Model file for the job. Use its own axes, mm. A direction names the side the tool comes from. Round coordinates to 2 decimals unless told otherwise and drop trailing zeros. Order: outer loops, then holes, each group sorted by start corner. A loop starts at its lowest first (then second) coordinate and runs counter-clockwise, first axis right, second up. Notation, with made-up numbers: (53, -38.75) - (62, -38.75) arc R23 cw to (62, -14.75) - close; hole circle Ø11 at (-24, 52.5). An arc over 180 degrees is marked (long way). Answer as CSV lines item,"result". Start each with the question number.
1. Band-saw the part on A-A on x = -4.75. List the corners of the cut face in (y, z), then the cut area to 3 significant figures.
2. Pull direction Y, two halves, no side cores. Call faces 1 (the face through (10.3, -7.1, 1.4)), 2 (the face through (11.27, -5.35, 1.4)), 3 (the face through (-4.95, 8.69, 1.4)): released by +Y, released by -Y, zero draft, split by the parting line, or undercut.
3. Wall check: line 1 along Y through (x, z) = (-0.65, 80); line 2 along Z through (x, y) = (0.8, -12.5); line 3 along X through (y, z) = (-11, 52.5). Give the ranges that are in metal, low to high. Write a range as [from, to].
4. Pin check, flat tips, straight feed: pin 1 Ø2.5 at (y, z) = (-12.5, 0) entering from +X; pin 2 Ø1.6 at (y, z) = (-12.5, 40) entering from +X; pin 3 Ø4 at (x, z) = (3.5, 74.5) entering from +Y; pin 4 Ø4 at (y, z) = (12.5, 29.5) entering from -X. Stop position of each tip, or through.
5. 3-axis set-ups, long thin cutter, end or side, ignore diameter. For faces 4 (the face through (11.04, -5.796, 1.4)), 5 (the face through (11.27, 5.35, 1.4)), 6 (the face through (0.5, -12.5, 1.4)): which of +Z, -Z, +X, -X, +Y, -Y reach the whole face in a straight line?
```python
from build123d import *

# Parameters (mm, degrees)
SKETCH1_R           = 10
BOSS_EXTRUDE1_DEPTH = 100
SKETCH4_W           = 0.5
SKETCH4_H           = 15
BOSS_EXTRUDE3_DEPTH = 200
CIRPATTERN7_COUNT   = 6
SKETCH7_R           = 1
CUT_EXTRUDE2_DEPTH  = 5
CIRPATTERN9_COUNT   = 6


with BuildPart() as part:
    # Sketch1 → Boss-Extrude1 (new, symmetric)
    with BuildSketch(Plane.XY):
        Circle(SKETCH1_R)
    extrude(amount=BOSS_EXTRUDE1_DEPTH, both=True)

    # Sketch4 → Boss-Extrude3 (add)
    with BuildSketch(Plane.XY.offset(100)):
        with Locations((-0.75, 7.5)):
            Rectangle(SKETCH4_W, SKETCH4_H)
        with Locations((0.75, 7.5)):
            Rectangle(SKETCH4_W, SKETCH4_H)
    boss_extrude3 = extrude(amount=-BOSS_EXTRUDE3_DEPTH)

    # CirPattern7: Boss-Extrude3 ×6 about axis
    cirpattern7_axis = Axis((0, 0, 0), (0, 0, 1))
    for i in range(1, CIRPATTERN7_COUNT):
        add(boss_extrude3.rotate(cirpattern7_axis, i * 360 / CIRPATTERN7_COUNT))

    # Sketch7 → Cut-Extrude2 (cut)
    with BuildSketch(Plane.ZY.offset(1)):
        with Locations((-80, 12.5)):
            Circle(SKETCH7_R)
        with Locations((-40, 12.5)):
            Circle(SKETCH7_R)
        with Locations((0, 12.5)):
            Circle(SKETCH7_R)
        with Locations((40, 12.5)):
            Circle(SKETCH7_R)
        with Locations((80, 12.5)):
            Circle(SKETCH7_R)
    cut_extrude2 = extrude(amount=-CUT_EXTRUDE2_DEPTH, mode=Mode.SUBTRACT)

    # CirPattern9: Cut-Extrude2 ×6 about axis
    cirpattern9_axis = Axis((0, 0, 100), (0, 0, 1))
    for i in range(1, CIRPATTERN9_COUNT):
        add(cut_extrude2.rotate(cirpattern9_axis, i * 360 / CIRPATTERN9_COUNT), mode=Mode.SUBTRACT)


solid = part.part
```
Reply:
1,outline,"(-8.8, -100) - (8.8, -100) - (8.8, 100) - (-8.8, 100) - close"
1,area,"3,520 mm2"
2,face 1,"released by -Y"
2,face 2,"undercut"
2,face 3,"released by +Y"
3,line 1,"y = [-15, -13.5], [-11.5, 11.5], [13.5, 15]"
3,line 2,"z = [-100, -81], [-79, -41], [-39, -1], [1, 39], [41, 79], [81, 100]"
3,line 3,"x = [-1, -0.5], [0.5, 1]"
4,pin 1,"stops at x = 1"
4,pin 2,"passes through"
4,pin 3,"stops at y = 9.89"
4,pin 4,"stops at x = -1"
5,face 4,"+Z, -Z"
5,face 5,"+Z, -Z, +X"
5,face 6,"+Z, -Z, -Y"
